Here's the drawing with two shaded views (mm, measured from the low corner). I have some questions. Coordinates: 2 decimals unless noted, no trailing zeros. Write each loop counter-clockwise with the first axis right and the second up, starting at its lowest first coordinate (ties: lowest second). Pieces come first, ordered by that corner, then holes.
Item 1: If we section it at A-A (z = 25): Please give me the cut outline in (x, y), then the cut area to 3 significant figures.
Item 2: If I drill on line 1 (X direction, y = 2.35, z = 25); line 2 (X direction, y = 1.75, z = 27.5), over which ranges is the centre line in solid material (lowest first)?
Item 3: We'd pull the mould along Y, two halves only. Please class the marked faces 1 and 2: +Y half, -Y half, draft (parallel to the pull), parting line (faces both ways), or undercut.
Item 4: If we section it at B-B (x = 20): Please give me the cut outline in (y, z), then the cut area to 3 significant figures.
Item 5: I'm going to push flat-ended pins straight in: pin 1 Ø5 at (x, z) = (20, 25) entering from +Y (3 decimals); pin 2 Ø5 at (x, z) = (17.14, 43.28) entering from +Y. Where does each tip first touch, or does it pass through?
Item 6: If we section it at C-C (y = 2.45): Please give me the cut outline in (x, z), then the cut area to 3 significant figures.
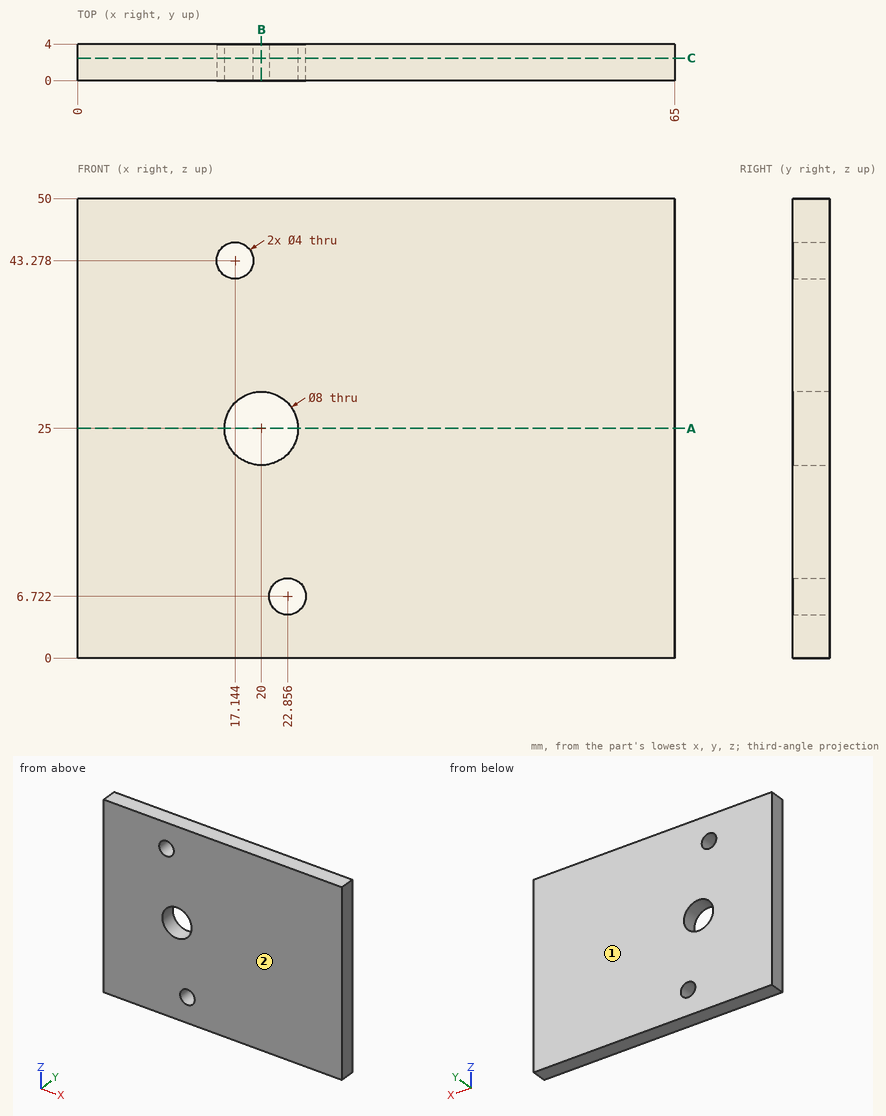
Answer list:
1. outline: (0, 0) - (16, 0) - (16, 4) - (0, 4) - close; (24, 0) - (65, 0) - (65, 4) - (24, 4) - close
1. area: 228 mm2
2. line 1: x = 0 to 16, 24 to 65
2. line 2: x = 0 to 16.88, 23.12 to 65
3. face 1: +Y half
3. face 2: -Y half
4. outline: (0, 0) - (4, 0) - (4, 21) - (0, 21) - close; (0, 29) - (4, 29) - (4, 50) - (0, 50) - close
4. area: 168 mm2
5. pin 1: passes through
5. pin 2: stops at y = 4
6. outline: (0, 0) - (65, 0) - (65, 50) - (0, 50) - close; hole circle Ø4 at (17.14, 43.28); hole circle Ø8 at (20, 25); hole circle Ø4 at (22.86, 6.72)
6. area: 3,170 mm2
